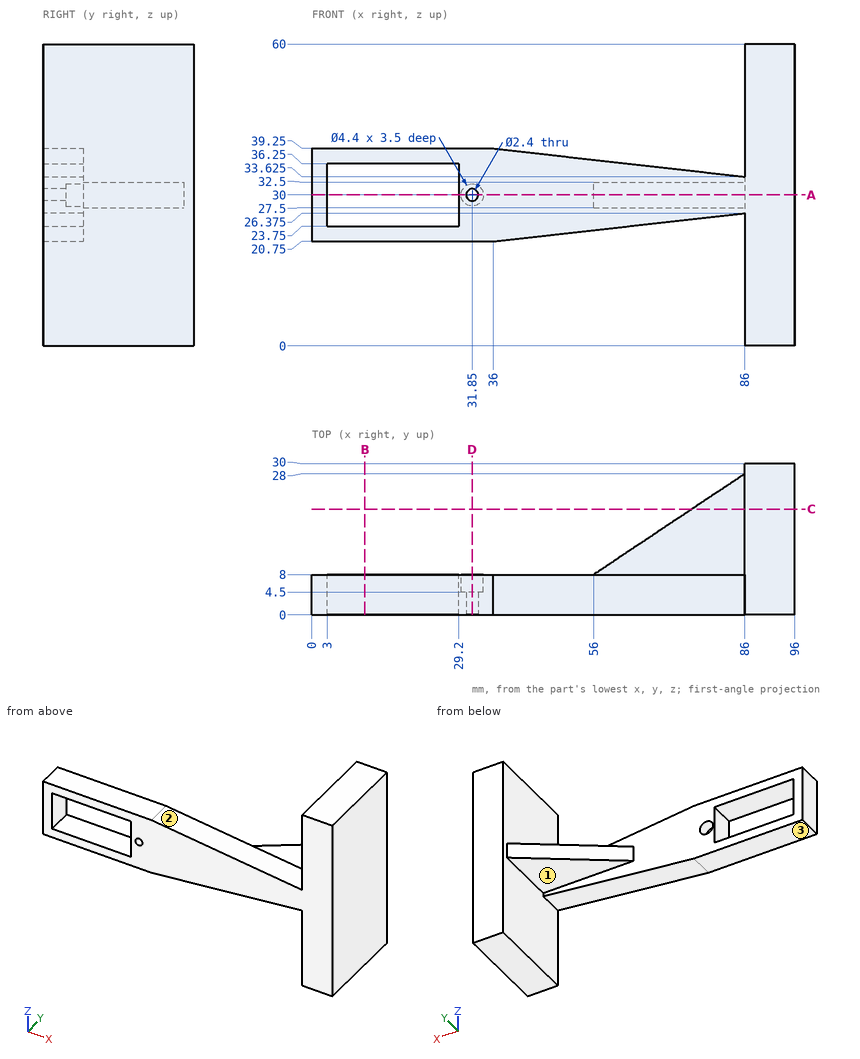
Job drawing, mm, ordinate dimensions from the low corner. One solid piece. A direction names the side the tool comes from. Coordinates: 2 decimals unless noted, no trailing zeros. Order: outer loops, then holes, each group sorted by start corner. A loop starts at its lowest first (then second) coordinate and runs counter-clockwise, first axis right, second up. Notation, with made-up numbers: (2, -40) - (54, -40) arc R26 ccw to (54, -14) - close; hole circle Ø9 at (44.5, -4.5). An arc over 180 degrees is marked (long way). Return JSON: item names as keys, results as strings. Group by question number.
1) Flat gauge pins, fed straight in: P1, Ø6.5, axis at x = 13.5, y = 2.5, coming from the -Z side; P2, Ø8, axis at x = 28.5, z = 29, coming from the +Y side; P3, Ø4, axis at x = 19, y = 4.5, coming from the +Z side. Where does each tip first touch, or does it go through?
2) Saw through at B-B, the plane x = 10.5. Write the cut outline in (y, z).
3) Saw through at A-A, the plane z = 30. Write the cut outline in (x, y), plus the area to 3 significant figures.
4) Saw through at D-D, the plane x = 31.85. Write the cut outline in (y, z), plus the area to 3 significant figures.
5) Tool access for the marked faces 1, 2 and 3: list every direction of +Z, -Z, +X, -X, +Y, -Y with a clear straight run to the whole face (end or side of a thin tool).
6) Saw through at C-C, the plane y = 21. Write the cut outline in (x, z).
7) Probe line 1 (X direction, y = 2.35, z = 30); line 2 (Z direction, x = 18, y = 5); line 3 (X direction, y = 23, z = 38). List the from-to ranges inside material, lowest first. Write a range as from..to.
Values found:
{
 "1": {"P1": "stops at z = 20.75", "P2": "stops at y = 8", "P3": "stops at z = 39.25"},
 "2": {"outline": "(0, 20.75) - (8, 20.75) - (8, 23.75) - (0, 23.75) - close; (0, 36.25) - (8, 36.25) - (8, 39.25) - (0, 39.25) - close"},
 "3": {"outline": "(0, 0) - (3, 0) - (3, 8) - (0, 8) - close; (29.2, 0) - (30.65, 0) - (30.65, 4.5) - (29.65, 4.5) - (29.65, 8) - (29.2, 8) - close; (33.05, 0) - (96, 0) - (96, 30) - (86, 30) - (86, 28) - (56, 8) - (34.05, 8) - (34.05, 4.5) - (33.05, 4.5) - close", "area": "1,050 mm²"},
 "4": {"outline": "(0, 20.75) - (8, 20.75) - (8, 27.8) - (4.5, 27.8) - (4.5, 28.8) - (0, 28.8) - close; (0, 31.2) - (4.5, 31.2) - (4.5, 32.2) - (8, 32.2) - (8, 39.25) - (0, 39.25) - close", "area": "122 mm²"},
 "5": {"face 1": "-Z, -X, +Y", "face 2": "+Z, +Y, -Y", "face 3": "-Z, -X, +Y, -Y"},
 "6": {"outline": "(75.5, 27.5) - (86, 27.5) - (86, 0) - (96, 0) - (96, 60) - (86, 60) - (86, 32.5) - (75.5, 32.5) - close"},
 "7": {"line 1": "x = 0..3, 29.2..30.65, 33.05..96", "line 2": "z = 20.75..23.75, 36.25..39.25", "line 3": "x = 86..96"}
}
